Source: CAD feature listing. Evaluate the final solid. Frame: model axes, mm. Face numbers are marked on the shaded views. Give positions to 0.01 mm unless a question says otherwise; leave off trailing zeros. Order: outer loops, then holes, each group sorted by start corner. A loop starts at its lowest first (then second) coordinate and runs counter-clockwise, first axis right, second up. Notation, with made-up numbers: M 24,36.5 L 73,36.5 A25 cw 73,61.5 Z; hole C -19,43.25 d7. An arc over 180 degrees is marked long. Answer in a Markdown table with one row per item. Add a question column.
(1) Material intervals for line 1 along X through (y, z) = (57, 16.5); line 2 along X through (y, z) = (13.5, 15.75); line 3 along X through (y, z) = (42, 18), sorted ascending.
(2) Pin query (flat end, axial travel): P1, Ø7, axis at x = 37.5, z = 14.5, coming from the +Y side; P2, Ø3, axis at y = 44, z = 15.5, coming from the -X side; P3, Ø3, axis at x = 87.5, z = 17, coming from the +Y side. Return the tip coordinate at first contact, or that it passes through.
(3) Section query B-B, the plane x = 65.5. Return loops of the section in (y, z), plus the area to 3 significant figures.
(4) Section query C-C, the plane y = 34. Return loops of the section in (x, z), plus the area to 3 significant figures.
(5) Mould query, pull axis X, two halves, no side actions, for the marked faces 1, 2 and 3. Classes: pulls with the +X half, pulls with the -X half, needs draft (parallel to the pull), parting line crosses it, or undercut.
(6) Section query D-D, the plane z = 10.25. Return loops of the section in (x, y).
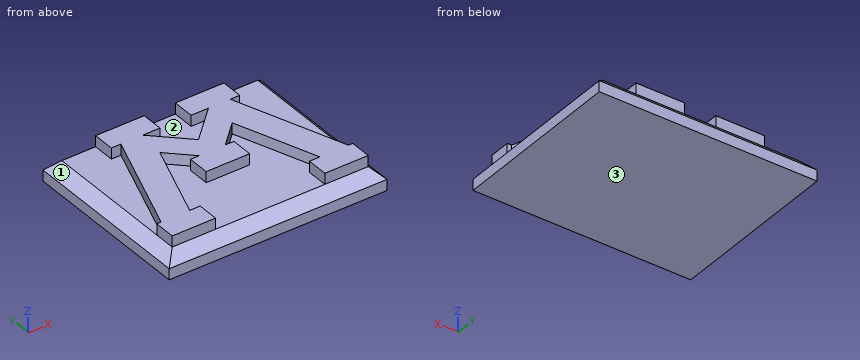
from build123d import *

# Parameters (mm, degrees)
F0_W     = 127
F0_H     = 101.6
F1_DEPTH = 12.7
F2_SIZE  = 6.35
F4_DEPTH = 6.35


with BuildPart() as f1:
    # F0 (on Top) → F1 (new body)
    with BuildSketch(Plane.XY):
        with Locations((63.5, 50.8)):
            Rectangle(F0_W, F0_H)
    extrude(amount=F1_DEPTH)

    # F2
    f2_edges = [f1.edges().sort_by_distance(p)[0] for p in [
        (0, 50.8, 12.7),
        (63.5, 101.6, 12.7),
        (127, 50.8, 12.7),
        (63.5, 0, 12.7),
    ]]
    chamfer(f2_edges, length=F2_SIZE)

    # F3 (on face) → F4 (join)
    with BuildSketch(Plane.XY.offset(12.7)):
        Polygon((82.67119, 82.55), (63.5, 64.081497), (44.32881, 82.55), (54.423093, 82.55), (54.423093, 95.25), (26.081875, 95.25), (26.081875, 82.55), (31.62881, 82.55), (8.904249, 18.794981), (6.35, 18.794981), (6.35, 6.35), (31.62881, 6.35), (31.62881, 18.794981), (25.537017, 18.794981), (42.386614, 66.067462), (55.88, 53.068654), (50.8, 53.068654), (50.8, 40.368654), (76.2, 40.368654), (76.2, 53.068654), (71.12, 53.068654), (84.613386, 66.067462), (101.462983, 18.794981), (95.37119, 18.794981), (95.37119, 6.35), (120.65, 6.35), (120.65, 18.794981), (118.095751, 18.794981), (95.37119, 82.55), (100.918125, 82.55), (100.918125, 95.25), (72.576907, 95.25), (72.576907, 82.55), align=None)
    extrude(amount=F4_DEPTH)


solid = f1.part
Values follow:
| question | item | result |
|---|---|---|
| 1 | line 1 | x = 22.52 to 39.15, 51.8 to 75.2, 87.85 to 104.48 |
| 1 | line 2 | x = 6.35 to 31.63, 95.37 to 120.65 |
| 1 | line 3 | x = 17.18 to 33.81, 50.8 to 76.2, 93.19 to 109.82 |
| 2 | P1 | stops at y = 96.95 |
| 2 | P2 | stops at x = 17.35 |
| 2 | P3 | stops at y = 95.25 |
| 3 | outline | M 0,0 L 101.6,0 L 101.6,6.35 L 95.25,12.7 L 66.01,12.7 L 66.01,19.05 L 40.37,19.05 L 40.37,12.7 L 6.35,12.7 L 0,6.35 Z |
| 3 | area | 1,410 mm² |
| 4 | outline | M 0,0 L 127,0 L 127,6.35 L 120.65,12.7 L 112.68,12.7 L 112.68,19.05 L 96.04,19.05 L 96.04,12.7 L 30.96,12.7 L 30.96,19.05 L 14.32,19.05 L 14.32,12.7 L 6.35,12.7 L 0,6.35 Z |
| 4 | area | 1,780 mm² |
| 5 | face 1 | pulls with the -X half |
| 5 | face 2 | undercut |
| 5 | face 3 | needs draft |
| 6 | outline | M 3.9,3.9 L 123.1,3.9 L 123.1,97.7 L 3.9,97.7 Z |
